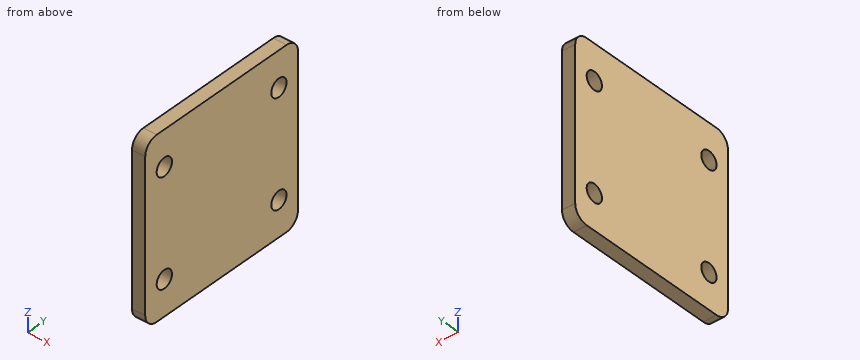
```python
from build123d import *

# Parameters (mm, degrees)
SKETCH1_W           = 40
SKETCH1_H           = 40
BOSS_EXTRUDE1_DEPTH = 3
FILLET1_R           = 3
CUT_EXTRUDE1_REACH  = 5
SKETCH2_R           = 2


with BuildPart() as part:
    # Sketch1 → Boss-Extrude1 (new body)
    with BuildSketch(Plane.ZY.offset(26.051745534)):
        with Locations((-36.163138966, 1200.261717599)):
            Rectangle(SKETCH1_W, SKETCH1_H)
    extrude(amount=BOSS_EXTRUDE1_DEPTH)

    # Fillet1
    fillet1_edges = [part.edges().sort_by_distance(p)[0] for p in [
        (-27.551745534, 1220.261717599, -56.163138966),
        (-27.551745534, 1220.261717599, -16.163138966),
        (-27.551745534, 1180.261717599, -16.163138966),
        (-27.551745534, 1180.261717599, -56.163138966),
    ]]
    fillet(fillet1_edges, radius=FILLET1_R)

    # Sketch2 → Cut-Extrude1 (cut, up to next)
    with BuildSketch(Plane.ZY.offset(29.051745534), mode=Mode.PRIVATE) as cut_extrude1_sk1:
        with Locations((-48.163138966, 1215.261717599)):
            Circle(SKETCH2_R)
    cut_extrude1_tool1 = extrude(cut_extrude1_sk1.sketch, amount=-CUT_EXTRUDE1_REACH, mode=Mode.PRIVATE) & part.part
    add(cut_extrude1_tool1.solids().sort_by_distance((-29.051746, 1215.261718, -48.163139))[0], mode=Mode.SUBTRACT)
    # Sketch2 → Cut-Extrude1 (cut, up to next)
    with BuildSketch(Plane.ZY.offset(29.051745534), mode=Mode.PRIVATE) as cut_extrude1_sk2:
        with Locations((-24.163138966, 1215.261717599)):
            Circle(SKETCH2_R)
    cut_extrude1_tool2 = extrude(cut_extrude1_sk2.sketch, amount=-CUT_EXTRUDE1_REACH, mode=Mode.PRIVATE) & part.part
    add(cut_extrude1_tool2.solids().sort_by_distance((-29.051746, 1215.261718, -24.163139))[0], mode=Mode.SUBTRACT)
    # Sketch2 → Cut-Extrude1 (cut, up to next)
    with BuildSketch(Plane.ZY.offset(29.051745534), mode=Mode.PRIVATE) as cut_extrude1_sk3:
        with Locations((-24.163138966, 1185.261717599)):
            Circle(SKETCH2_R)
    cut_extrude1_tool3 = extrude(cut_extrude1_sk3.sketch, amount=-CUT_EXTRUDE1_REACH, mode=Mode.PRIVATE) & part.part
    add(cut_extrude1_tool3.solids().sort_by_distance((-29.051746, 1185.261718, -24.163139))[0], mode=Mode.SUBTRACT)
    # Sketch2 → Cut-Extrude1 (cut, up to next)
    with BuildSketch(Plane.ZY.offset(29.051745534), mode=Mode.PRIVATE) as cut_extrude1_sk4:
        with Locations((-48.163138966, 1185.261717599)):
            Circle(SKETCH2_R)
    cut_extrude1_tool4 = extrude(cut_extrude1_sk4.sketch, amount=-CUT_EXTRUDE1_REACH, mode=Mode.PRIVATE) & part.part
    add(cut_extrude1_tool4.solids().sort_by_distance((-29.051746, 1185.261718, -48.163139))[0], mode=Mode.SUBTRACT)


solid = part.part
```
Part model, mm, in its own coordinate system. Round coordinates to 2 decimals unless told otherwise and drop trailing zeros. Write each loop counter-clockwise with the first axis right and the second up, starting at its lowest first coordinate (ties: lowest second). Pieces come first, ordered by that corner, then holes. Notation, with made-up numbers: M -21.75,81.5 L 19.25,81.5 A28 cw 19.25,102.5 Z; hole C 66.5,-12 d2. An arc over 180 degrees is marked long. One line per question, with ' | ' between items.
(1) Saw through at A-A on z = -24.5. Write the cut outline in (x, y), then the cut area to 3 significant figures.
Answer key:
outline: M -29.05,1180.26 L -26.05,1180.26 L -26.05,1183.29 L -29.05,1183.29 Z; M -29.05,1187.23 L -26.05,1187.23 L -26.05,1213.29 L -29.05,1213.29 Z; M -29.05,1217.23 L -26.05,1217.23 L -26.05,1220.26 L -29.05,1220.26 Z | area: 96.3 mm^2
(2) Probe line 1 along Z through (x, y) = (-28.8, 1217); line 2 along Y through (x, z) = (-27.1, -22.5); line 3 along Y through (x, z) = (-27.35, -54). List the from-to ranges inside material, lowest first.
Answer key:
line 1: z = -56.16 to -49.15, -47.17 to -25.15, -23.17 to -16.16 | line 2: y = 1180.26 to 1184.15, 1186.37 to 1214.15, 1216.37 to 1220.26 | line 3: y = 1180.38 to 1220.14
(3) Saw through at B-B on x = -27.3. Write the cut outline in (y, z), then the cut area to 3 significant figures.
Answer key:
outline: M 1180.26,-53.16 A3 ccw 1183.26,-56.16 L 1217.26,-56.16 A3 ccw 1220.26,-53.16 L 1220.26,-19.16 A3 ccw 1217.26,-16.16 L 1183.26,-16.16 A3 ccw 1180.26,-19.16 Z; hole C 1185.26,-48.16 d4; hole C 1185.26,-24.16 d4; hole C 1215.26,-48.16 d4; hole C 1215.26,-24.16 d4 | area: 1,540 mm^2
